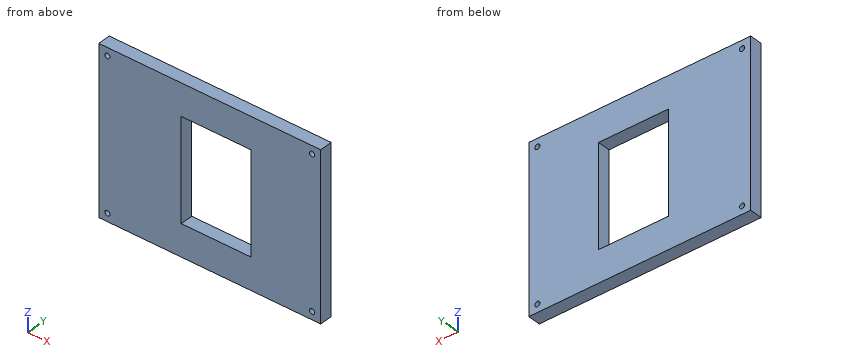
Autodesk Fusion 360 part; units mm, degrees
sketch "Sketch1" plane through (0, 0, 0) normal (0, 1, 0) x (1, 0, 0)
  line L0 (0, 0) -> (350, 0)
  line L1 (350, 0) -> (350, -260)
  line L2 (350, -260) -> (0, -260)
  line L3 (0, -260) -> (0, 0)
  circle A0 centre (13.5555, -247.4318) radius 4.05
  line L4 (175, -260) -> (175, 0) construction
  line L5 (0, -130) -> (350, -130) construction
  line L6 (350, -130) -> (0, -130) construction
  circle A1 centre (336.4445, -247.4318) radius 4.05
  circle A2 centre (336.4445, -12.5682) radius 4.05
  circle A3 centre (13.5555, -12.5682) radius 4.05
  line L7 (40, -260) -> (40.238, -260)
  line L8 (130, -50) -> (240, -50)
  line L9 (130, -50) -> (130, -210)
  line L10 (130, -210) -> (240, -210)
  line L11 (240, -210) -> (240, -50)
  dimension "d1" = 350
  dimension "d2" = 260
  dimension "d3" = 8.1
extrude "Extrude1" add sketch "Sketch1" along normal blind 20
For this review, take the finished solid that the model builds, in its own axes (mm). Coordinates: 2 decimals unless noted, no trailing zeros. Write each loop counter-clockwise with the first axis right and the second up, starting at its lowest first coordinate (ties: lowest second). Pieces come first, ordered by that corner, then holes. Notation, with made-up numbers: (19, 80) -> (66, 80) arc R3 cw to (66, 85) -> close; hole circle Ø4 at (-8, 38). An arc over 180 degrees is marked (long way). Put each result on its own line as item: value.
Q1. Wall thickness on L1, parallel to X at y = 10, z = 149; L2, parallel to Z at x = 173.5, y = 2: over which ranges is each line inside the solid? List them lowest first.
From the geometry:
L1: x = 0 to 130, 240 to 350
L2: z = 0 to 50, 210 to 260
Q2. Take a section at B-B, the plane y = 6.5. State the section outline as (x, z) points, then the cut area to 3 significant figures.
From the geometry:
outline: (0, 0) -> (350, 0) -> (350, 260) -> (0, 260) -> close; hole circle Ø8.1 at (13.56, 12.57); hole circle Ø8.1 at (13.56, 247.43); hole (130, 50) -> (240, 50) -> (240, 210) -> (130, 210) -> close; hole circle Ø8.1 at (336.44, 12.57); hole circle Ø8.1 at (336.44, 247.43)
area: 73,200 mm2
Q3. Take a section at A-A, the plane z = 73. State the section outline as (x, y) points, then the cut area to 3 significant figures.
From the geometry:
outline: (0, 0) -> (130, 0) -> (130, 20) -> (0, 20) -> close; (240, 0) -> (350, 0) -> (350, 20) -> (240, 20) -> close
area: 4,800 mm2
